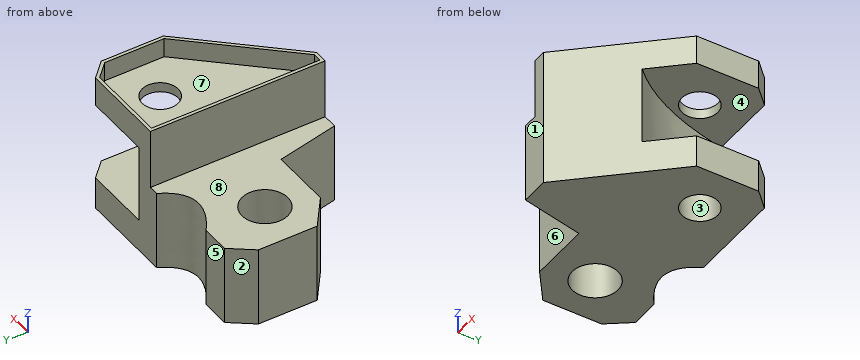
from build123d import *

# Parameters (mm, degrees)
BOSS_EXTRUDE1_DEPTH     = 43
SKETCH2_R               = 7
CUT_EXTRUDE1_DEPTH      = 43
SKETCH3_R               = 5.5
CUT_EXTRUDE2_DEPTH      = 43
CUT_EXTRUDE3_DEPTH      = 81.267405813
CUT_EXTRUDE3_DEPTH_BACK = 81.267405813
SKETCH4_W               = 43.989032816
SKETCH4_H               = 19
SKETCH5_W               = 35.072240015
SKETCH5_H               = 24
CUT_EXTRUDE4_DEPTH      = 43
BOSS_EXTRUDE2_DEPTH     = 24
CUT_EXTRUDE5_DEPTH      = 6


with BuildPart() as part:
    # Sketch1 → Boss-Extrude1 (new body)
    with BuildSketch(Plane.XY):
        with BuildLine():
            Line((0, 0), (-9.330406061, 7))
            Line((-9.330406061, 7), (-9.330406061, 25))
            Line((-9.330406061, 25), (-4.078758954, 32))
            Line((-4.078758954, 32), (4.669593939, 32))
            add(Edge.make_bspline(
                [(4.669593939, 32), (17.970448987, 22.058553501), (24.343418505, 34.49495508)],
                knots=[0, 0, 0, 1, 1, 1], degree=2))
            Line((24.343418505, 34.49495508), (53.343418505, 34.49495508))
            Line((53.343418505, 34.49495508), (58.343418505, 29.49495508))
            Line((58.343418505, 29.49495508), (58.343418505, 10.49495508))
            Line((58.343418505, 10.49495508), (31.309807425, -19))
            Line((31.309807425, -19), (22.799304213, -19))
            Line((22.799304213, -19), (18.70656591, 0))
            Line((18.70656591, 0), (0, 0))
        make_face()
    extrude(amount=BOSS_EXTRUDE1_DEPTH)

    # Sketch2 → Cut-Extrude1 (cut)
    with BuildSketch(Plane(origin=(0, 0, 0), x_dir=(-1, 0, 0), z_dir=(0, 0, -1))):
        with Locations((-4.669593939, 14)):
            Circle(SKETCH2_R)
    extrude(amount=-CUT_EXTRUDE1_DEPTH, mode=Mode.SUBTRACT)

    # Sketch3 → Cut-Extrude2 (cut)
    with BuildSketch(Plane.XY.offset(43)):
        with Locations((44.343418505, 20.49495508)):
            Circle(SKETCH3_R)
    extrude(amount=-CUT_EXTRUDE2_DEPTH, mode=Mode.SUBTRACT)

    # Sketch4 → Cut-Extrude3 (cut, two sides: drawn at the far end of the back side and taken through both)
    with BuildSketch(Plane(origin=(0, 0, 0), x_dir=(1, 0, 0), z_dir=(0, 1, 0)).offset(-CUT_EXTRUDE3_DEPTH_BACK)):
        with Locations((5.245897655, -34.002948031)):
            Rectangle(SKETCH4_W, SKETCH4_H)
    extrude(amount=CUT_EXTRUDE3_DEPTH + CUT_EXTRUDE3_DEPTH_BACK, mode=Mode.SUBTRACT)

    # Sketch5 → Cut-Extrude4 (cut)
    with BuildSketch(Plane(origin=(0, 0, 0), x_dir=(1, 0, 0), z_dir=(0, 1, 0))):
        with Locations((50.243902929, -22)):
            Rectangle(SKETCH5_W, SKETCH5_H)
    extrude(amount=CUT_EXTRUDE4_DEPTH, mode=Mode.SUBTRACT)

    # Sketch6 → Boss-Extrude2 (add)
    with BuildSketch(Plane.XY.offset(10)):
        with BuildLine():
            Line((32.707782921, 34.49495508), (32.707782921, 0))
            Line((32.707782921, 0), (48.724263868, 0))
            add(Edge.make_bspline(
                [(48.724263868, 0), (39.533647592, 9.345830828), (35.169336989, 21.979196109), (32.707782921, 34.49495508)],
                knots=[0, 0, 0, 0, 1, 1, 1, 1], degree=3))
        make_face()
    extrude(amount=BOSS_EXTRUDE2_DEPTH)

    # 3DSketch1 → Cut-Extrude5 (cut)
    with BuildSketch(Plane(origin=(30.869867984, -18, 43), x_dir=(0.39376955076248915, 0.9192091932157269, 0), z_dir=(0, 0, 1))):
        Polygon((0, 0), (36.9748267, -12.961129751), (53.701528522, -5.795768579), (56.020931318, 0), (46.299237224, 22.694163546), (-1.035398889, 2.417018217), align=None)
    extrude(amount=-CUT_EXTRUDE5_DEPTH, mode=Mode.SUBTRACT)


solid = part.part
Input: part model. Units: mm. Frame: model coordinates. Face numbers are marked on the shaded views. A direction names the side the tool comes from. Coordinates: 2 decimals unless noted, no trailing zeros. Loops run counter-clockwise (first coordinate to the right, second up) from the corner with the lowest first, then second, coordinate; pieces in that order, holes last.
Q1. Cut plane B-B (x = 52). Output: boundary loops of the cut face in (y, z).
Q2. Cut plane A-A (z = 39.5). Output: boundary loops of the cut face in (x, y).
Q3. Draft query along Y for the marked faces 1, 2 and 3. Return one class per face: +Y half, -Y half, draft (parallel to the pull), parting line (faces both ways), or undercut.
Q4. Cut plane C-C (y = -3). Output: boundary loops of the cut face in (x, z), then the cut area to 3 significant figures.
Q5. Cut plane D-D (x = 43). Give the number of separate pieces and of enclosed holes in the cut face, then the cut area to 3 significant figures.
Q6. Contact query for flat-ended pins moving along their axis: pin 1 (5.5 mm diameter, centred on y = -5.5, z = 32, fed in from -X); pin 2 (4 mm diameter, centred on x = 4, z = 14.5, fed in from +Y); pin 3 (7.5 mm diameter, centred on x = 41.5, y = 14, fed in from +Z). Output: stop coordinate, or through.
Q7. Set-up query: the marked faces 4, 5, 6, 7 and 8. Return all of +Z, -Z, +X, -X, +Y, -Y with unobstructed straight access to the full face (end or side cutting, diameter ignored); none if empty.
Q8. Material intervals for line 1 (Z direction, x = 50, y = 21); line 2 (Z direction, x = -3, y = 22); line 3 (X direction, y = 6, z = 41), sorted ascending.
Working result:
1. outline: (3.57, 0) - (34.49, 0) - (34.49, 10) - (3.57, 10) - close; (3.57, 34) - (34.49, 34) - (34.49, 43) - (33.49, 43) - (33.49, 37) - (5.05, 37) - (5.05, 43) - (3.57, 43) - close
2. outline: (27.24, -19) - (31.31, -19) - (58.34, 10.49) - (58.34, 29.49) - (53.34, 34.49) - (27.24, 34.49) - close; hole (28.24, -18) - (30.87, -18) - (57.34, 10.88) - (57.34, 29.08) - (52.93, 33.49) - (28.24, 33.49) - close
3. face 1: -Y half
3. face 2: +Y half
3. face 3: undercut
4. outline: (19.35, 0) - (45.97, 0) - (45.97, 43) - (44.62, 43) - (44.62, 37) - (28.24, 37) - (28.24, 43) - (27.24, 43) - (27.24, 24.5) - (19.35, 24.5) - close
4. area: 901 mm2
5. separate pieces: 3
5. enclosed holes: 0
5. area: 726 mm2
6. pin 1: stops at x = 27.24
6. pin 2: stops at y = 32
6. pin 3: stops at z = 37
7. face 4: +X, +Y
7. face 5: +Z, -Z, -X, +Y
7. face 6: +Z, -Z, -X, -Y
7. face 7: +Z
7. face 8: +Z, -X, +Y, -Y
8. line 1: z = 0 to 10, 34 to 37
8. line 2: z = 0 to 24.5
8. line 3: x = 27.24 to 28.24, 52.87 to 54.22
